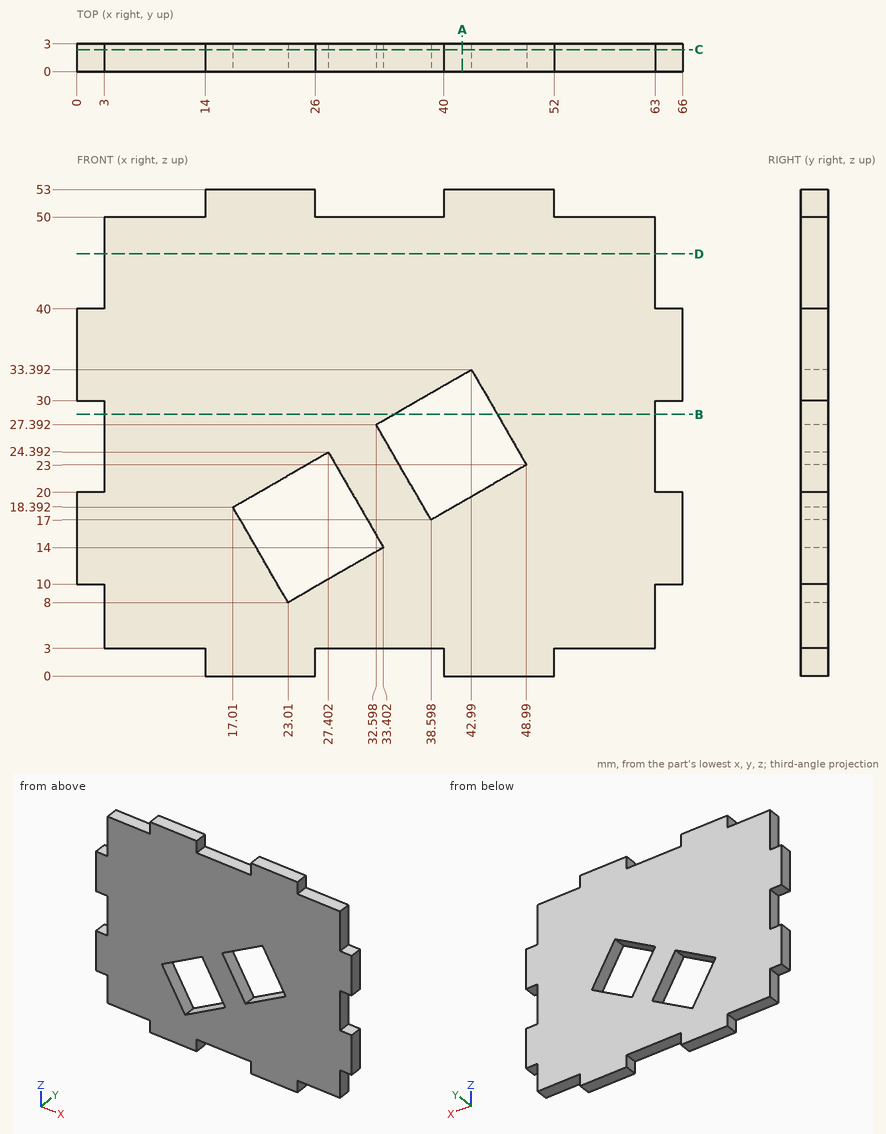
Print and shaded views of the part. All mm, measured from the part's lowest x, y and z. Round coordinates to 2 decimals unless told otherwise and drop trailing zeros. Write each loop counter-clockwise with the first axis right and the second up, starting at its lowest first coordinate (ties: lowest second). Pieces come first, ordered by that corner, then holes. Notation, with made-up numbers: (53, 39.5) -> (100, 39.5) arc R29 ccw to (100, 71.5) -> close; hole circle Ø6 at (-26, 24). An arc over 180 degrees is marked (long way). Write item = value, one per line.
(1) Band-saw the part on A-A (x = 42). Give the cut face in (y, z).
Answer:
outline = (0, 0) -> (3, 0) -> (3, 18.96) -> (0, 18.96) -> close; (0, 32.82) -> (3, 32.82) -> (3, 53) -> (0, 53) -> close
(2) Band-saw the part on B-B (z = 28.5). Give the cut face in (x, y) (1 decimal), then the cut area to 3 significant figures.
Answer:
outline = (3, 0) -> (34.5, 0) -> (34.5, 3) -> (3, 3) -> close; (45.8, 0) -> (63, 0) -> (63, 3) -> (45.8, 3) -> close
area = 146 mm2
(3) Flat gauge pins, fed straight in: pin 1 (1.5 mm diameter, centred on y = 1, z = 24.5, fed in from +X); pin 2 (1 mm diameter, centred on y = 2, z = 28, fed in from -X); pin 3 (1.5 mm diameter, centred on y = 1, z = 1.5, fed in from +X). Where does each tip first touch, or does it go through?
Answer:
pin_1 = 63
pin_2 = 3
pin_3 = 52
(4) Band-saw the part on C-C (y = 2.4). State how many separate pieces and enclosed holes the cut face has, then the cut area to 3 significant figures.
Answer:
separate_pieces = 1
enclosed_holes = 2
area = 2,800 mm2
(5) Probe L1, parallel to Z at x = 63.5, y = 2.4; L2, parallel to Z at x = 58, y = 1.45; L3, parallel to X at y = 2.35, z = 46. List the from-to ranges inside material, lowest first.
Answer:
L1 = 10 to 20, 30 to 40
L2 = 3 to 50
L3 = 3 to 63
(6) Band-saw the part on D-D (z = 46). Give the cut face in (x, y), then the cut area to 3 significant figures.
Answer:
outline = (3, 0) -> (63, 0) -> (63, 3) -> (3, 3) -> close
area = 180 mm2
